```python
from build123d import *

# Parameters (mm, degrees)
SKETCH1_R           = 3.8
BOSS_EXTRUDE1_DEPTH = 7


with BuildPart() as part:
    # Sketch1 → Boss-Extrude1 (new body)
    with BuildSketch(Plane(origin=(0, 0, 0), x_dir=(1, 0, 0), z_dir=(0, 1, 0))):
        with Locations(Location((0, 0, 0), (0, 0, 270))):
            Circle(SKETCH1_R)
        with BuildLine():
            Line((1.5, -1.2), (2.7, -1.2))
            Line((2.7, -1.2), (2.7, 1.2))
            Line((2.7, 1.2), (1.5, 1.2))
            ThreePointArc((1.5, 1.2), (1.287867966, 1.287867966), (1.2, 1.5))
            Line((1.2, 1.5), (1.2, 2.7))
            Line((1.2, 2.7), (-1.2, 2.7))
            Line((-1.2, 2.7), (-1.2, 1.5))
            ThreePointArc((-1.2, 1.5), (-1.287867966, 1.287867966), (-1.5, 1.2))
            Line((-1.5, 1.2), (-2.7, 1.2))
            Line((-2.7, 1.2), (-2.7, -1.2))
            Line((-2.7, -1.2), (-1.5, -1.2))
            ThreePointArc((-1.5, -1.2), (-1.287867966, -1.287867966), (-1.2, -1.5))
            Line((-1.2, -1.5), (-1.2, -2.7))
            Line((-1.2, -2.7), (1.2, -2.7))
            Line((1.2, -2.7), (1.2, -1.5))
            ThreePointArc((1.2, -1.5), (1.287867966, -1.287867966), (1.5, -1.2))
        make_face(mode=Mode.SUBTRACT)
    extrude(amount=BOSS_EXTRUDE1_DEPTH)


solid = part.part
```
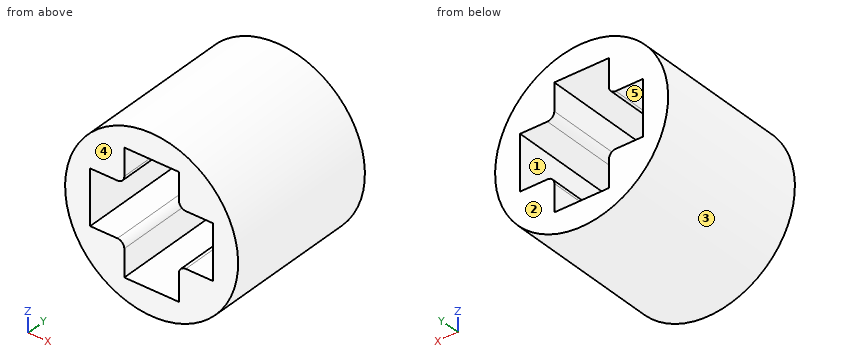
Build history of the part. All positions in model axes, mm. Face numbers are marked on the shaded views. A direction names the side the tool comes from. Coordinates: 2 decimals unless noted, no trailing zeros. Order: outer loops, then holes, each group sorted by start corner. A loop starts at its lowest first (then second) coordinate and runs counter-clockwise, first axis right, second up.
Item 1: Saw through at B-B on z = 0. List the corners of the cut face in (x, y).
Filled in:
outline: (-3.8, 0) - (-2.7, 0) - (-2.7, 7) - (-3.8, 7) - close; (2.7, 0) - (3.8, 0) - (3.8, 7) - (2.7, 7) - close
Item 2: Mould opens along Z. For the marked faces 1, 2 and 3 say: released by +Z, released by -Z, zero draft, split by the parting line, or undercut.
Filled in:
face 1: undercut
face 2: zero draft
face 3: split by the parting line
Item 3: Tool access for the marked faces 4 and 5: list every direction of +Z, -Z, +X, -X, +Y, -Y with a clear straight run to the whole face (end or side of a thin tool).
Filled in:
face 4: +Z, -Z, +X, -X, -Y
face 5: +Y, -Y
Item 4: Saw through at D-D on z = 3. List the corners of the cut face in (x, y), then the cut area to 3 significant figures.
Filled in:
outline: (-2.33, 0) - (2.33, 0) - (2.33, 7) - (-2.33, 7) - close
area: 32.7 mm2
Item 5: Drop flat-ended pins along their axis: pin 1 Ø1 at (y, z) = (4, 2.5) entering from -X; pin 2 Ø1.3 at (x, y) = (-2, 2.5) entering from -Z; pin 3 Ø3 at (y, z) = (5, 3) entering from -X; pin 4 Ø2 at (x, z) = (0.5, 0.5) entering from +Y. Give the stop position or say it passes through.
Filled in:
pin 1: stops at x = -3.23
pin 2: stops at z = -3.55
pin 3: stops at x = -3.49
pin 4: passes through
Item 6: Saw through at C-C on y = 0.5. List the corners of the cut face in (x, z), then the cut area to 3 significant figures.
Filled in:
outline: circle Ø7.6 at (0, 0); hole (-2.7, -1.2) - (-1.5, -1.2) arc R0.3 cw to (-1.2, -1.5) - (-1.2, -2.7) - (1.2, -2.7) - (1.2, -1.5) arc R0.3 cw to (1.5, -1.2) - (2.7, -1.2) - (2.7, 1.2) - (1.5, 1.2) arc R0.3 cw to (1.2, 1.5) - (1.2, 2.7) - (-1.2, 2.7) - (-1.2, 1.5) arc R0.3 cw to (-1.5, 1.2) - (-2.7, 1.2) - close
area: 25.1 mm2
Item 7: Drill centre lines: L1, parallel to Z at x = -1, y = 2.25; L2, parallel to Z at x = 1.5, y = 6; L3, parallel to X at y = 2.5, z = 0.75. Where is each one in solid material? Low to high.
Filled in:
L1: z = -3.67 to -2.7, 2.7 to 3.67
L2: z = -3.49 to -1.2, 1.2 to 3.49
L3: x = -3.73 to -2.7, 2.7 to 3.73
Item 8: Saw through at A-A on x = 0. List the corners of the cut face in (y, z).
Filled in:
outline: (0, -3.8) - (7, -3.8) - (7, -2.7) - (0, -2.7) - close; (0, 2.7) - (7, 2.7) - (7, 3.8) - (0, 3.8) - close
